Geometry: see drawing. Coordinates: mm, zero at the bounding-box minimum. A direction names the side the tool comes from. Give positions to 0.01 mm unless a question says otherwise; leave off trailing zeros. Write each loop counter-clockwise with the first axis right and the second up, starting at its lowest first coordinate (ties: lowest second). Pieces come first, ordered by that corner, then holes. Notation, with made-up numbers: M -22,27.5 L 4,27.5 A26 ccw 4,66.5 Z; hole C 58,58 d5. An arc over 180 degrees is marked long. Use one line per item in the form item = value. Start each with the question number.
Item 1: Access query for the marked faces 4 and 5. Directions: +Z, -Z, +X, -X, +Y, -Y. A direction counts if a zero-diameter tool reaches every point of the face in a straight line with its end or side. Return the directions, or none.
Item 2: Section query C-C on x = 2.25. Return loops of the section in (y, z), then the cut area to 3 significant figures.
Item 3: Section query D-D on z = 5.5. Return loops of the section in (x, y).
Item 4: Section query B-B on z = 2.25. Return loops of the section in (x, y).
Item 5: Section query A-A on y = 6.5. Return loops of the section in (x, z), then the cut area to 3 significant figures.
Item 6: Pull-direction query (X, two-part tool) for the marked faces 1, 2 and 3; classes: released by +X, released by -X, zero draft, split by the parting line, or undercut.
Item 7: Material intervals for line 1 along X through (y, z) = (13.5, 3.25); line 2 along Y through (x, z) = (8.5, 2.5); line 3 along Y through (x, z) = (3.5, 9.25), sorted ascending. Write a range as from..to.
Item 8: Contact query for flat-ended pins moving along their axis: P1, Ø3.5, axis at x = 16.5, z = 5.5, coming from the +Y side; P2, Ø2, axis at x = 1.5, z = 7.5, coming from the +Y side. Output: stop coordinate, or through.
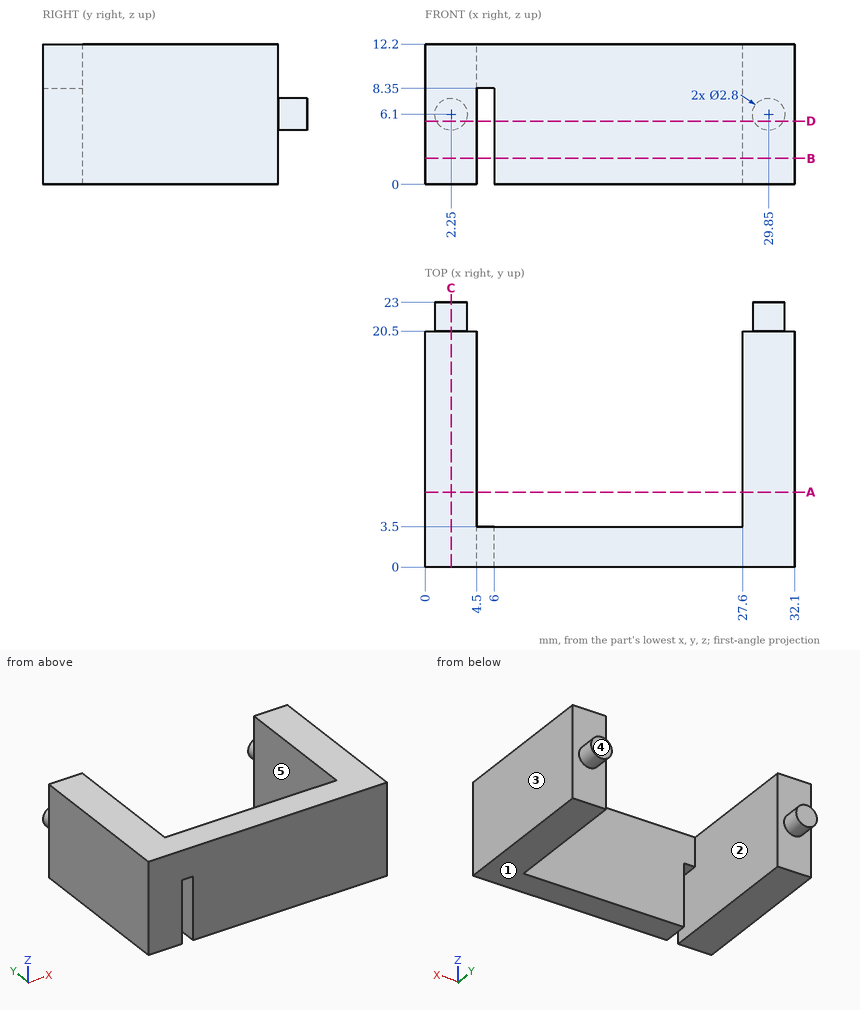
Answer sheet:
q1.face_4 = +Z, -Z, +X, -X, +Y
q1.face_5 = +Z, -Z, +Y
q2.outline = M 0,0 L 20.5,0 L 20.5,4.7 L 23,4.7 L 23,7.5 L 20.5,7.5 L 20.5,12.2 L 0,12.2 Z
q2.area = 257 mm2
q3.outline = M 0,0 L 4.5,0 L 4.5,20.5 L 3.51,20.5 L 3.51,23 L 0.99,23 L 0.99,20.5 L 0,20.5 Z; M 6,0 L 32.1,0 L 32.1,20.5 L 31.11,20.5 L 31.11,23 L 28.59,23 L 28.59,20.5 L 27.6,20.5 L 27.6,3.5 L 6,3.5 Z
q4.outline = M 0,0 L 4.5,0 L 4.5,20.5 L 0,20.5 Z; M 6,0 L 32.1,0 L 32.1,20.5 L 27.6,20.5 L 27.6,3.5 L 6,3.5 Z
q5.outline = M 0,0 L 4.5,0 L 4.5,12.2 L 0,12.2 Z; M 27.6,0 L 32.1,0 L 32.1,12.2 L 27.6,12.2 Z
q5.area = 110 mm2
q6.face_1 = zero draft
q6.face_2 = undercut
q6.face_3 = released by +X
q7.line_1 = 0..4.5, 27.6..32.1
q7.line_2 = 0..3.5
q7.line_3 = 0..20.5
q8.P1 = 3.5
q8.P2 = 23
